The model under review builds one solid part; all positions refer to its coordinate system, in mm. Round coordinates to 2 decimals unless told otherwise and drop trailing zeros. Order: outer loops, then holes, each group sorted by start corner. A loop starts at its lowest first (then second) coordinate and runs counter-clockwise, first axis right, second up.
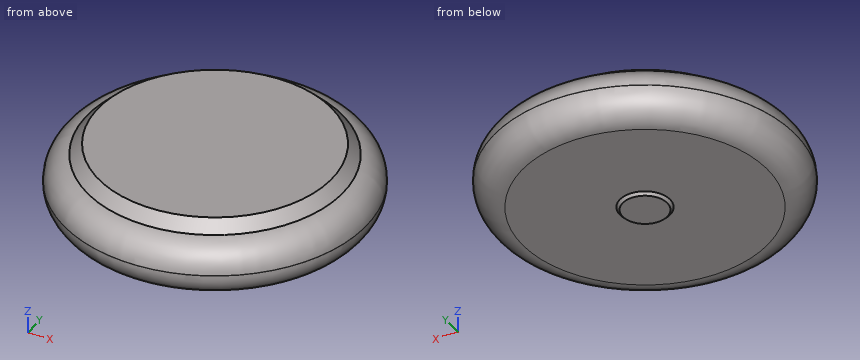
```python
from build123d import *

# Parameters (mm, degrees)
SKETCH1_R           = 108
BOSS_EXTRUDE1_DEPTH = 40
SKETCH3_R           = 91.518206512
BOSS_EXTRUDE3_DEPTH = 8
CHAMFER1_SIZE       = 8
FILLET2_R           = 20
SKETCH5_R           = 20
BOSS_EXTRUDE4_DEPTH = 2
CHAMFER2_SIZE       = 4


# Some blends are built 0.0001 mm under size
with BuildPart() as part:
    # Sketch1 → Boss-Extrude1 (new body)
    with BuildSketch(Plane.XY):
        Circle(SKETCH1_R)
    extrude(amount=BOSS_EXTRUDE1_DEPTH)

    # Sketch3 → Boss-Extrude3 (add)
    with BuildSketch(Plane.XY.offset(40)):
        Circle(SKETCH3_R)
    extrude(amount=BOSS_EXTRUDE3_DEPTH)

    # Chamfer1
    chamfer1_edges = [part.edges().sort_by_distance(p)[0] for p in [
        (-91.518206512, 0, 48),
    ]]
    chamfer(chamfer1_edges, length=CHAMFER1_SIZE - 0.0001)  # a hair under: the kernel refuses the full size

    # Fillet2
    # the kernel refuses this fillet: 20 mm, written as the material it takes off along each edge
    with BuildSketch(Plane(origin=(0, 0, 0), x_dir=(1, 0, 0), z_dir=(0, -1, 0))) as fillet2_piece_1:
        with BuildLine():
            CenterArc((108 - FILLET2_R, FILLET2_R), FILLET2_R, 270, 90)
            Line((108 - FILLET2_R, 0), (108 - FILLET2_R, -FILLET2_R * 0.02))
            Line((108 - FILLET2_R, -FILLET2_R * 0.02), (108 + FILLET2_R * 0.02, -FILLET2_R * 0.02))
            Line((108 + FILLET2_R * 0.02, -FILLET2_R * 0.02), (108 + FILLET2_R * 0.02, FILLET2_R))
            Line((108 + FILLET2_R * 0.02, FILLET2_R), (108, FILLET2_R))
        make_face()
    revolve(axis=Axis((0, 0, 0), (0, 0, 1)), mode=Mode.SUBTRACT)
    with BuildSketch(Plane(origin=(0, 0, 40), x_dir=(1, 0, 0), z_dir=(0, -1, 0))) as fillet2_piece_2:
        with BuildLine():
            CenterArc((88, -19.688123906), FILLET2_R, 0, 79.868362225)
            Line((108, -19.688123906), (108.4, -19.688123906))
            Line((108.4, -19.688123906), (108.4, 0))
            Line((108.4, 0), (108, 0.4))
            ThreePointArc((108, 0.4), (99.759103256, 0.4), (91.588570642, 0.393762478))
            Line((91.588570642, 0.393762478), (91.518206512, 0))
        make_face()
    revolve(axis=Axis((0, 0, 40), (0, 0, 1)), mode=Mode.SUBTRACT)

    # Sketch5 → Boss-Extrude4 (add)
    with BuildSketch(Plane(origin=(0, 0, 0), x_dir=(-1, 0, 0), z_dir=(0, 0, -1))):
        with Locations(Location((0, 0, 0), (0, 0, 180))):
            Circle(SKETCH5_R)
    extrude(amount=BOSS_EXTRUDE4_DEPTH)

    # Chamfer2
    # the kernel refuses this chamfer: 4 mm, written as the material it takes off along each edge
    with BuildSketch(Plane(origin=(0, 0, -2), x_dir=(1, 0, 0), z_dir=(0, 1, 0))) as chamfer2_piece_1_section:
        Polygon((20, -CHAMFER2_SIZE), (20 - CHAMFER2_SIZE, 0), (20, 0), align=None)
    chamfer2_piece_1 = revolve(axis=Axis((0, 0, -2), (0, 0, -1)), mode=Mode.PRIVATE)
    chamfer2_piece_1 = split(chamfer2_piece_1, bisect_by=Plane(origin=(-17.007894049, 0, 0), z_dir=(0, 0, -1)), keep=Keep.TOP, mode=Mode.PRIVATE)
    add(chamfer2_piece_1, mode=Mode.SUBTRACT)


solid = part.part
```
(1) Consider section D-D (z = 14). Write out the cut boundary in (x, y), and give its area (3 significant figures).
Data:
outline: circle Ø214.16 at (0, 0)
area: 36,000 mm2
(2) Consider section C-C (z = 37.5). Write out the cut boundary in (x, y), and give its area (3 significant figures).
Data:
outline: circle Ø196.45 at (0, 0)
area: 30,300 mm2
(3) Insertion check: pin 1 (1 mm diameter, centred on y = -24.5, z = 27, fed in from +X); pin 2 (12 mm diameter, centred on x = -14.5, z = 16.5, fed in from +Y); pin 3 (1.5 mm diameter, centred on x = -41.5, z = 23.5, fed in from +Y). Each pin has a flat end and moves straight along its axis. Give the tip position at first contact, or say it passes through.
Data:
pin 1: stops at x = 104.21
pin 2: stops at y = 107.6
pin 3: stops at y = 99.77
(4) To check wall thickness, follow probe 1 along Z at (x, y) = (-45, 4); probe 2 along Y at (x, z) = (-20, 29); probe 3 along Y at (x, z) = (-18, 27). State the ranges of each line that lie inside material, in increasing order.
Data:
probe 1: z = 0 to 48
probe 2: y = -104.11 to 104.11
probe 3: y = -105.32 to 105.32
